from build123d import *

# Parameters (mm, degrees)
F1_DEPTH = 13.1826
F3_D     = 2.54
F5_D     = 2.54


with BuildPart() as f1:
    # F0 (on Front) → F1 (new body, symmetric)
    with BuildSketch(Plane.XZ):
        Polygon((-22.04417, 16.991249), (-31.56917, 16.991249), (-31.56917, -17.933751), (0.70153, -17.933751), (0.70153, -8.408751), (-22.04417, -8.408751), align=None)
    extrude(amount=F1_DEPTH, both=True)

    # F3 (through all)
    with Locations(Plane.XY.offset(-8.408751)):
        with Locations((-5.88977, 6.5913), (-5.88977, -6.5913)):
            Hole(F3_D / 2)

    # F5 (through all)
    with Locations(Plane.YZ.offset(-22.04417)):
        with Locations((-6.5913, 4.62864), (6.5913, 4.62864)):
            Hole(F5_D / 2)


solid = f1.part
Geometry check sheet. Reference: the model listing, model coordinates, mm. A direction names the side the tool comes from. Give positions to 0.01 mm unless a question says otherwise; leave off trailing zeros. Loops run counter-clockwise (first coordinate to the right, second up) from the corner with the lowest first, then second, coordinate; pieces in that order, holes last. Notation, with made-up numbers: (43, 3) -> (60, 3) arc R33 cw to (60, 39) -> close; hole circle Ø5 at (62.5, -7.75). An arc over 180 degrees is marked (long way). Answer in a Markdown table with one row per item. Add a question column.
1) Cross-section at C-C on z = 0.5. Record the boundary of the cut face in (x, y), and give its area (3 significant figures).
2) Cross-section at B-B on x = -6.5. Record the boundary of the cut face in (y, z).
3) Draft check along Z on faces 1 (the face through (-23, -13.183, -4)), 2 (the face through (-16, 0, -17.934)), 3 (the face through (-26.87, 5.38, 5.01)), 4 (the face through (-11, 0, -8.409)). Enter one of: pulls with the +Z half, pulls with the -Z half, needs draft (parallel to the pull), parting line crosses it, or undercut.
4) Material ranges on probe 1 along Z at (x, y) = (-14.5, -8); probe 2 along Z at (x, y) = (-28, 6); probe 3 along X at (y, z) = (6.75, 11), recorded low to high. Write a range as from..to.
5) Set-up check for faces 5 (the face through (-22.044, 0, 4)), 6 (the face through (-31.569, 0, 0)): record each of +Z, -Z, +X, -X, +Y, -Y from which the full face is reachable in a straight line by a thin tool's end or side.
6) Cross-section at D-D on x = -13. Record the boundary of the cut face in (y, z).
7) Gauge pin test, flat ends, axial feed: P1, Ø7, axis at x = -12, y = -4.5, coming from the +Z side; P2, Ø4, axis at y = -6.59, z = 4.63, coming from the -X side; P3, Ø4, axis at y = 9, z = 0, coming from the +X side. Record the tip position at first contact, or that the pin passes through.
8) Cross-section at A-A on y = 8.75. Record the boundary of the cut face in (x, z), and give its area (3 significant figures).
Outcome:
| question | item | result |
|---|---|---|
| 1 | outline | (-31.57, -13.18) -> (-22.04, -13.18) -> (-22.04, 13.18) -> (-31.57, 13.18) -> close |
| 1 | area | 251 mm^2 |
| 2 | outline | (-13.18, -17.93) -> (-7.71, -17.93) -> (-7.71, -8.41) -> (-13.18, -8.41) -> close; (-5.48, -17.93) -> (5.48, -17.93) -> (5.48, -8.41) -> (-5.48, -8.41) -> close; (7.71, -17.93) -> (13.18, -17.93) -> (13.18, -8.41) -> (7.71, -8.41) -> close |
| 3 | face 1 | needs draft |
| 3 | face 2 | pulls with the -Z half |
| 3 | face 3 | undercut |
| 3 | face 4 | pulls with the +Z half |
| 4 | probe 1 | z = -17.93..-8.41 |
| 4 | probe 2 | z = -17.93..3.5, 5.75..16.99 |
| 4 | probe 3 | x = -31.57..-22.04 |
| 5 | face 5 | +Z, +X, +Y, -Y |
| 5 | face 6 | +Z, -Z, -X, +Y, -Y |
| 6 | outline | (-13.18, -17.93) -> (13.18, -17.93) -> (13.18, -8.41) -> (-13.18, -8.41) -> close |
| 7 | P1 | stops at z = -8.41 |
| 7 | P2 | stops at x = -31.57 |
| 7 | P3 | stops at x = -22.04 |
| 8 | outline | (-31.57, -17.93) -> (0.7, -17.93) -> (0.7, -8.41) -> (-22.04, -8.41) -> (-22.04, 16.99) -> (-31.57, 16.99) -> close |
| 8 | area | 549 mm^2 |
